Can you work these out from the model? Positions are in its coordinate system, mm. Face numbers are marked on the shaded views. A direction names the side the tool comes from. Coordinates: 2 decimals unless noted, no trailing zeros. Order: outer loops, then holes, each group sorted by start corner. A loop starts at its lowest first (then second) coordinate and runs counter-clockwise, first axis right, second up. Notation, with made-up numbers: M -12.75,54.5 L 23.25,54.5 A12 cw 23.25,72.5 Z; hole C 24,7 d3. An arc over 180 degrees is marked long. Answer as CSV lines item,"result". Start each with the question number.
1. If we mould it in two halves opening along Y, with no side actions, what happens to the marked faces 1, 2 and 3? For each: released by +Y, released by -Y, zero draft, split by the parting line, or undercut.
2. If we section it at A-A (x = 10): List the corners of the cut face in (y, z) for me.
3. If we section it at B-B (y = 5): List the corners of the cut face in (x, z) for me.
4. On a 3-axis mill with a long thin cutter (end or side, diameter ignored), from which of +Z, -Z, +X, -X, +Y, -Y can I reach the whole of each face in a straight line? I mean the marked faces 4 and 5. Say none if no direction works.
5. I need wall thicknesses on line 1 along Y through (x, z) = (-6, 2.3); line 2 along X through (y, z) = (-4.5, 3.2); line 3 along X through (y, z) = (1.5, 1). Which ranges of each line are inside material? Lowest first, please. Write a range as from..to.
6. Will these pins go through, and if not, where does the flat tip stop? pin 1 (1.3 mm diameter, centred on x = 9.5, y = 10.5, fed in from +Z); pin 2 (5 mm diameter, centred on x = 17.5, y = 9, fed in from +Z).
7. If we section it at D-D (x = 17): List the corners of the cut face in (y, z) for me.
8. If we section it at C-C (z = 1.55): List the corners of the cut face in (x, y) for me.
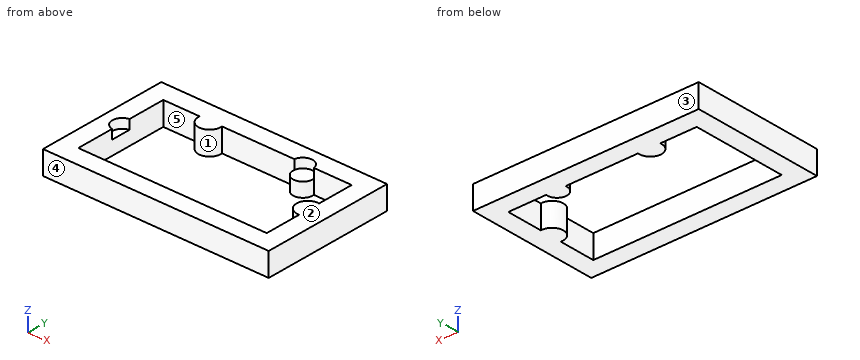
Autodesk Fusion 360 part; units mm, degrees
sketch "Sketch1" plane through (0, 0, 0) normal (0, 0, 1) x (1, 0, 0)
  line L0 (24.2, -14.2) -> (-24.2, -14.2)
  line L1 (-24.2, -14.2) -> (-24.2, 14.2)
  line L2 (-24.2, 14.2) -> (24.2, 14.2)
  line L3 (24.2, 14.2) -> (24.2, -14.2)
  line L4 (24.2, -14.2) -> (-24.2, 14.2) construction
  line L5 (-24.2, -14.2) -> (24.2, 14.2) construction
  dimension "d1" = 48.4
  dimension "d2" = 28.4
extrude "Extrude1" add sketch "Sketch1" along normal blind 5
shell "Shell1" thickness 4 removed faces 2 at (-8.0667, -4.7333, 5) at (-8.0667, -4.7333, 0)
sketch "Sketch2" plane through (0, 0, 5) normal (0, 0, 1) x (-1, 0, 0)
  line L0 (-20.2, -10.2) -> (-20.2, 10.2)
  line L1 (-20.2, 10.2) -> (20.2, 10.2)
  line L2 (20.2, 10.2) -> (20.2, -10.2)
  line L3 (20.2, -10.2) -> (-20.2, -10.2)
  line L4 (-24.2, -14.2) -> (24.2, -14.2)
  line L5 (24.2, -14.2) -> (24.2, 14.2)
  line L6 (24.2, 14.2) -> (-24.2, 14.2)
  line L7 (-24.2, 14.2) -> (-24.2, -14.2)
  circle A0 centre (19.9, 0) radius 2.1
  circle A1 centre (10, -9.9) radius 2.4
  circle A2 centre (-10, -9.9) radius 2.1
  circle A3 centre (-19.9, 0) radius 2.4
  line L8 (-20.2, 0) -> (20.2, 0) construction
  line L9 (0, -10.2) -> (0, 10.2) construction
  circle A4 centre (-10, 9.9) radius 2.1
  circle A5 centre (10, 9.9) radius 2.4
  dimension "d6" = 4.2
  dimension "d7" = 0.3
  dimension "d8" = 4.8
  dimension "d9" = 0.3
  dimension "d11" = 4.2
  dimension "d12" = 0.3
  dimension "d14" = 4.8
  dimension "d15" = 0.3
  dimension "d16" = 10
  dimension "d17" = 10
  dimension "d18" = 4.2
  dimension "d19" = 0.3
  dimension "d20" = 10
  dimension "d21" = 4.8
  dimension "d22" = 10
  dimension "d23" = 0.3
extrude "Extrude2" add sketch "Sketch2" against normal blind 5 contours L0 A3 | L3 A1 | L1 A5 picked at (-19.3318, 0.2231) picked at (10.663, -9.6523) picked at (10.5292, 10.7)
extrude "Extrude3" cut sketch "Sketch2" against normal blind 2 contours L3 A2 | L1 A4 | L2 A0 picked at (-9.6779, -10.88) picked at (-9.7428, 9.449) picked at (20.7929, -0.0996)
extrude "Extrude4" add sketch "Sketch2" against normal blind 3 from surface at -2 contours L3 A2 | L1 A4 | L2 A0 picked at (-9.4862, -9.6246) picked at (-10.1971, 10.7717) picked at (20.7929, -0.0996)
Solved:
1,face 1,"undercut"
1,face 2,"zero draft"
1,face 3,"released by +Y"
2,outline,"M -14.2,0 L -10.2,0 L -10.2,5 L -14.2,5 Z; M 7.8,0 L 14.2,0 L 14.2,5 L 12,5 L 12,3 L 7.8,3 Z"
3,outline,"M -24.2,0 L -20.2,0 L -20.2,5 L -24.2,5 Z; M 20.2,0 L 24.2,0 L 24.2,5 L 20.2,5 Z"
4,face 4,"+Z, -Z, +X, -X, -Y"
4,face 5,"+Z, -Z"
5,line 1,"-14.2..-10.2, 10.2..14.2"
5,line 2,"-24.2..-20.2, 20.2..24.2"
5,line 3,"-24.2..-20.2, 18.03..24.2"
6,pin 1,"z = 3"
6,pin 2,"z = 5"
7,outline,"M -14.2,0 L -10.2,0 L -10.2,5 L -14.2,5 Z; M 10.2,0 L 14.2,0 L 14.2,5 L 10.2,5 Z"
8,outline,"M -24.2,-14.2 L 24.2,-14.2 L 24.2,14.2 L -24.2,14.2 Z; hole M -20.2,-10.2 L 20.2,-10.2 L 20.2,-2.38 A2.4 cw long 20.2,2.38 L 20.2,10.2 L 12.08,10.2 A2.1 cw long 7.92,10.2 L -7.62,10.2 A2.4 cw long -12.38,10.2 L -20.2,10.2 Z"
